```python
from build123d import *

# Parameters (mm, degrees)
F1_DEPTH = 76.2
F3_DEPTH = 76.2
F5_DEPTH = 25.4


with BuildPart() as f1:
    # F0 (on Front) → F1 (new body)
    with BuildSketch(Plane.XZ):
        Polygon((35.288685, 50.8), (35.288685, 0), (187.688685, 0), (187.688685, 31.75), (117.838685, 31.75), (111.488685, 50.8), align=None)
    extrude(amount=F1_DEPTH)

    # F2 (on face) → F3 (cut)
    with BuildSketch(Plane.XZ.offset(76.2)):
        Polygon((82.892604, 50.8), (57.492604, 50.8), (57.492604, 38.1), (44.792604, 38.1), (44.792604, 25.4), (95.592604, 25.4), (95.592604, 38.1), (82.892604, 38.1), align=None)
    extrude(amount=-F3_DEPTH, mode=Mode.SUBTRACT)

    # F4 (on face) → F5 (cut)
    with BuildSketch(Plane.YZ.offset(187.688685)):
        Polygon((-62.926312, 14.859), (-50.8, 0), (-25.4, 0), (-12.126312, 14.859), align=None)
    extrude(amount=-F5_DEPTH, mode=Mode.SUBTRACT)


solid = f1.part
```
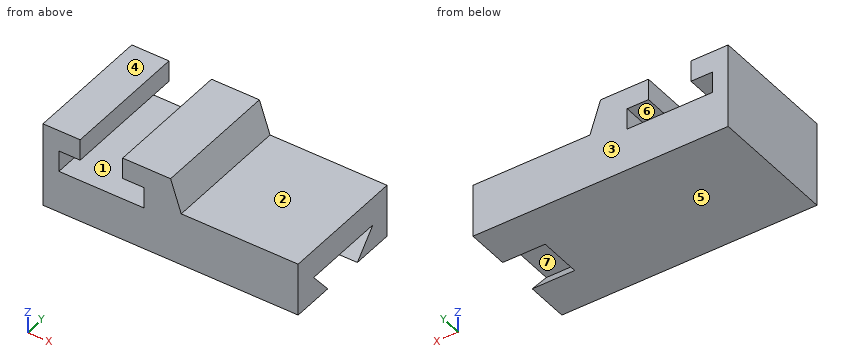
CAD build for the part. Positions are in the model's coordinates, mm. Face numbers are marked on the shaded views. A direction names the side the tool comes from. Round coordinates to 2 decimals unless told otherwise and drop trailing zeros. Write each loop counter-clockwise with the first axis right and the second up, starting at its lowest first coordinate (ties: lowest second). Pieces come first, ordered by that corner, then holes. Notation, with made-up numbers: (57, -3.75) - (91, -3.75) arc R22 ccw to (91, 19.25) - close; hole circle Ø6 at (77, -19.5). An arc over 180 degrees is marked (long way). Write item = value, one per line. Start each with the question number.
Q1. Probe L1, parallel to Z at x = 87, y = -58; L2, parallel to X at y = -73, z = 28; L3, parallel to X at y = -42, z = 9. List the from-to ranges inside material, lowest first. Write a range as from..to.
Q2. Band-saw the part on B-B (z = 27.5). Give the cut face in (x, y).
Q3. Drop flat-ended pins along their axis: pin 1 (6.5 mm diameter, centred on y = -48, z = 34.5, fed in from +X); pin 2 (4.5 mm diameter, centred on y = -43.5, z = 10.5, fed in from +X); pin 3 (10 mm diameter, centred on y = -21.5, z = 46, fed in from +X); pin 4 (15 mm diameter, centred on x = 72, y = -34, fed in from +Z). Give the stop position or say it passes through.
Q4. Band-saw the part on D-D (x = 176). Give the cut face in (y, z), then the cut area to 3 significant figures.
Q5. Which spindle directions (+Z, -Z, +X, -X, +Y, -Y) get a long thin tool onto all of the face, cutting with end or side? Do the marked faces 1, 2 and 3. Say none if no direction does.
Q6. Band-saw the part on C-C (y = -68). Give the cut face in (x, z), then the cut area to 3 significant figures.
Q7. Band-saw the part on A-A (x = 52). Give the cut face in (y, z), then the cut area to 3 significant figures.
Q8. Mould opens along Z. For the marked faces 4, 5, 6 and 7 say: pulls with the +Z half, pulls with the -Z half, needs draft (parallel to the pull), parting line crosses it, or undercut.
Answers below:
q1.L1 = 0..25.4, 38.1..50.8
q1.L2 = 35.29..44.79, 95.59..187.69
q1.L3 = 35.29..162.29
q2.outline = (35.29, -76.2) - (44.79, -76.2) - (44.79, 0) - (35.29, 0) - close; (95.59, -76.2) - (187.69, -76.2) - (187.69, 0) - (95.59, 0) - close
q3.pin_1 = 187.69
q3.pin_2 = 162.29
q3.pin_3 = 114.76
q3.pin_4 = 25.4
q4.outline = (-76.2, 0) - (-50.8, 0) - (-62.93, 14.86) - (-12.13, 14.86) - (-25.4, 0) - (0, 0) - (0, 31.75) - (-76.2, 31.75) - close
q4.area = 1,850 mm2
q5.face_1 = +Y, -Y
q5.face_2 = +Z, +X, +Y, -Y
q5.face_3 = +Z, -Z, +X, -X, +Y
q6.outline = (35.29, 0) - (187.69, 0) - (187.69, 31.75) - (117.84, 31.75) - (111.49, 50.8) - (82.89, 50.8) - (82.89, 38.1) - (95.59, 38.1) - (95.59, 25.4) - (44.79, 25.4) - (44.79, 38.1) - (57.49, 38.1) - (57.49, 50.8) - (35.29, 50.8) - close
q6.area = 5,380 mm2
q7.outline = (-76.2, 0) - (0, 0) - (0, 25.4) - (-76.2, 25.4) - close; (-76.2, 38.1) - (0, 38.1) - (0, 50.8) - (-76.2, 50.8) - close
q7.area = 2,900 mm2
q8.face_4 = pulls with the +Z half
q8.face_5 = pulls with the -Z half
q8.face_6 = undercut
q8.face_7 = undercut
